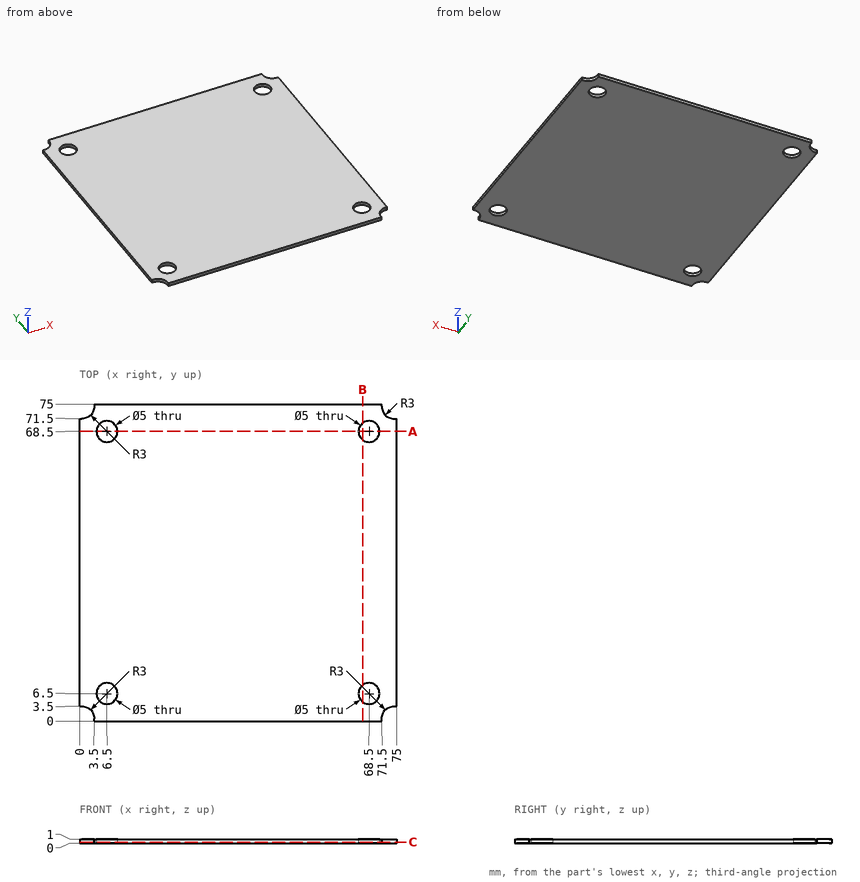
Design review of the part shown in the three views and the two pictorial views. Dimensions are in mm from the part's minimum x, y and z. Give positions to 0.01 mm unless a question says otherwise; leave off trailing zeros. Loops run counter-clockwise (first coordinate to the right, second up) from the corner with the lowest first, then second, coordinate; pieces in that order, holes last. Notation, with made-up numbers: M -30.75,14 L 21.25,14 A15 ccw 21.25,19 Z; hole C -36.5,69.25 d4. An arc over 180 degrees is marked long. Put each result on its own line as item: value. Start each with the question number.
(1) Add section A-A, the plane y = 68.5. Write out the cut boundary in (x, z), then the cut area to 3 significant figures.
(2) Wall thickness on L1, parallel to X at y = 68.5, z = 0.8; L2, parallel to Y at x = 69.5, z = 0.5: over which ranges is each line inside the solid? List them lowest first.
(3) For pin 1 (0.6 mm diameter, centred on x = 75, z = 0.5, fed in from -Y); pin 2 (0.6 mm diameter, centred on x = 74.5, z = 0.5, fed in from +Y), all flat-tipped, find the tip position at first contact; note any pin that passes through.
(4) Add section B-B, the plane x = 67. Write out the cut boundary in (y, z), then the cut area to 3 significant figures.
(5) Add section C-C, the plane z = 0.25. Write out the cut boundary in (x, y), then the cut area to 3 significant figures.
Result:
1. outline: M 0,0 L 4,0 L 4,1 L 0,1 Z; M 9,0 L 66,0 L 66,1 L 9,1 Z; M 71,0 L 75,0 L 75,1 L 71,1 Z
1. area: 65.0 mm^2
2. L1: x = 0 to 4, 9 to 66, 71 to 75
2. L2: y = 0 to 4.21, 8.79 to 66.21, 70.79 to 75
3. pin 1: stops at y = 3.5
3. pin 2: stops at y = 71.52
4. outline: M 0,0 L 4.5,0 L 4.5,1 L 0,1 Z; M 8.5,0 L 66.5,0 L 66.5,1 L 8.5,1 Z; M 70.5,0 L 75,0 L 75,1 L 70.5,1 Z
4. area: 67.0 mm^2
5. outline: M 0,3.5 L 0.5,3.5 A3 cw 3.5,0.5 L 3.5,0 L 71.5,0 L 71.5,0.5 A3 cw 74.5,3.5 L 75,3.5 L 75,71.5 L 74.5,71.5 A3 cw 71.5,74.5 L 71.5,75 L 3.5,75 L 3.5,74.5 A3 cw 0.5,71.5 L 0,71.5 Z; hole C 6.5,6.5 d5; hole C 6.5,68.5 d5; hole C 68.5,6.5 d5; hole C 68.5,68.5 d5
5. area: 5,510 mm^2
